Verification items for this drawing (mm, ordinates from the low corner). Round coordinates to 2 decimals unless told otherwise and drop trailing zeros. Loops run counter-clockwise (first coordinate to the right, second up) from the corner with the lowest first, then second, coordinate; pieces in that order, holes last. Notation, with made-up numbers: M -38.5,-24 L 3.5,-24 A20 ccw 3.5,3 Z; hole C 80.5,85.5 d5. An arc over 180 degrees is marked long. Write item = value, one per line. Start each with the question number.
(1) Cross-section at B-B on z = 48. Record the boundary of the cut face in (x, y).
(2) Cross-section at C-C on y = 6.75. Record the boundary of the cut face in (x, z), plus the area to 3 significant figures.
(3) Scan lines: L1, parallel to X at y = 5, z = 48; L2, parallel to X at y = 8.25, z = 35; L3, parallel to X at y = 7, z = 33.5. Record each from-to range of solid material in increasing order. Write a range as from..to.
(4) Cross-section at A-A on x = 48. Record the boundary of the cut face in (y, z).
(5) Cross-section at D-D on x = 35. Record the boundary of the cut face in (y, z), plus the area to 3 significant figures.
(6) Go/stop test with a flat-tipped pin: P1, Ø6.5, axis at x = 35, z = 35, coming from the +Y side. Record where the tip stops, or that it passes through.
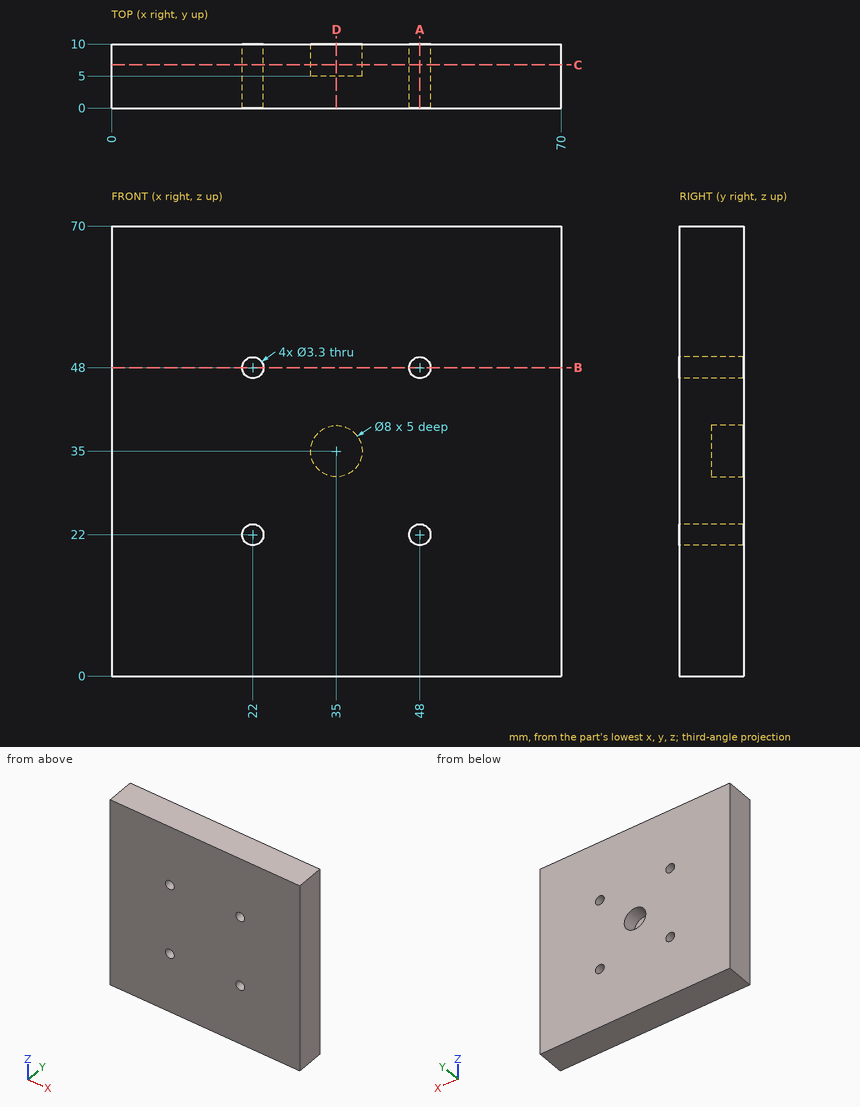
Result:
q1.outline = M 0,0 L 20.35,0 L 20.35,10 L 0,10 Z; M 23.65,0 L 46.35,0 L 46.35,10 L 23.65,10 Z; M 49.65,0 L 70,0 L 70,10 L 49.65,10 Z
q2.outline = M 0,0 L 70,0 L 70,70 L 0,70 Z; hole C 22,22 d3.3; hole C 22,48 d3.3; hole C 35,35 d8; hole C 48,22 d3.3; hole C 48,48 d3.3
q2.area = 4,820 mm^2
q3.L1 = 0..20.35, 23.65..46.35, 49.65..70
q3.L2 = 0..31, 39..70
q3.L3 = 0..31.29, 38.71..70
q4.outline = M 0,0 L 10,0 L 10,20.35 L 0,20.35 Z; M 0,23.65 L 10,23.65 L 10,46.35 L 0,46.35 Z; M 0,49.65 L 10,49.65 L 10,70 L 0,70 Z
q5.outline = M 0,0 L 10,0 L 10,31 L 5,31 L 5,39 L 10,39 L 10,70 L 0,70 Z
q5.area = 660 mm^2
q6.P1 = 5
